Check sheet for the drawn part. Datum: minimum x, y, z corner. Units: mm. Give positions to 0.01 mm unless a question says otherwise; leave off trailing zeros. Write each loop counter-clockwise with the first axis right and the second up, starting at its lowest first coordinate (ties: lowest second). Pieces come first, ordered by that corner, then holes. Notation, with made-up numbers: (62.25, 8.25) -> (93.25, 8.25) arc R32 cw to (93.25, 44.25) -> close; hole circle Ø8 at (80.5, -3). An arc over 180 degrees is marked (long way). Answer as CSV lines item,"result". Start each with the question number.
1) Sectioned sample at D-D on x = 51.5. Record the cut outline in (y, z).
2) Sectioned sample at C-C on z = 41. Record the cut outline in (x, y), and give its area (3 significant figures).
3) Sectioned sample at A-A on y = 0.4. Give the number of separate pieces and of enclosed holes in the cut face, and give its area (3 significant figures).
4) Sectioned sample at B-B on z = 85.2. Record the cut outline in (x, y).
5) Material ranges on L1, parallel to Z at x = 85.2, y = 0.75; L2, parallel to X at y = 0.4, z = 85.2; L3, parallel to Z at x = 37, y = 1.1 (1 decimal), recorded low to high.
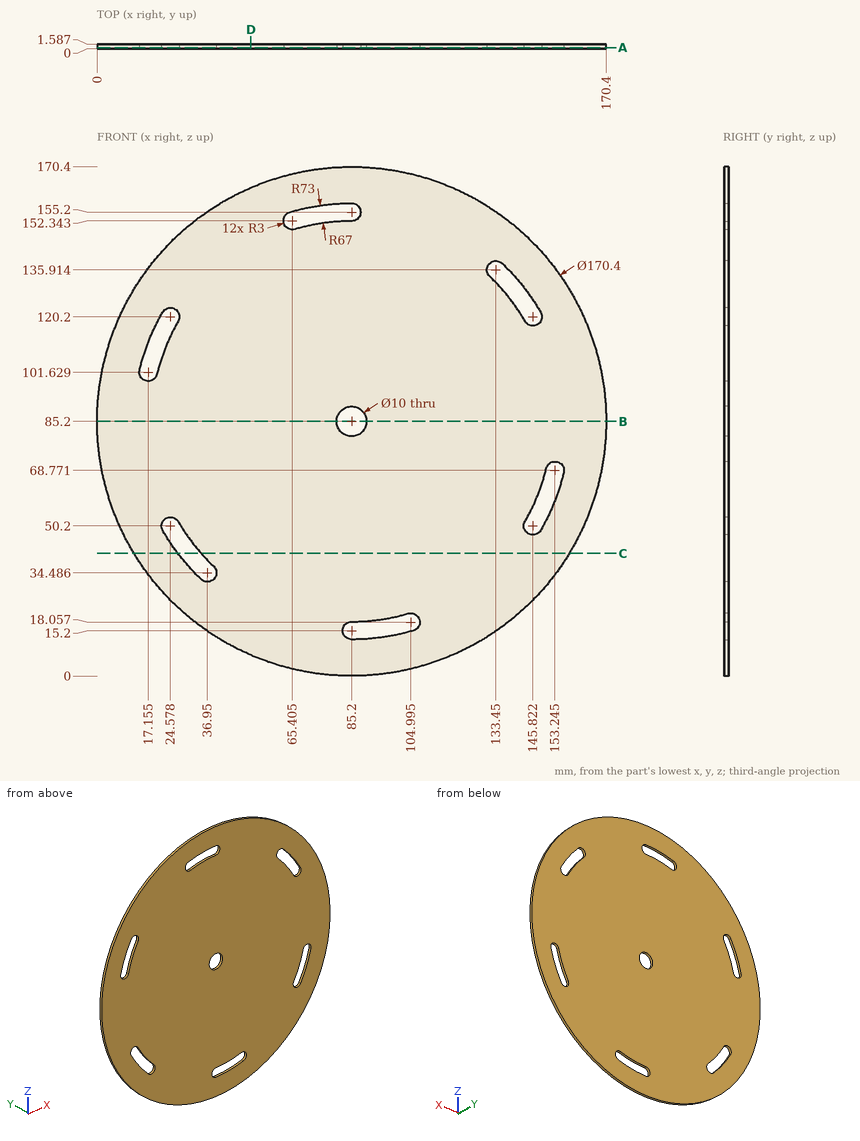
Ans:
1,outline,"(0, 6.95) -> (1.59, 6.95) -> (1.59, 163.45) -> (0, 163.45) -> close"
2,outline,"(12.36, 0) -> (27.1, 0) -> (27.1, 1.59) -> (12.36, 1.59) -> close; (34.85, 0) -> (158.04, 0) -> (158.04, 1.59) -> (34.85, 1.59) -> close"
2,area,"219 mm²"
3,separate pieces,"1"
3,enclosed holes,"7"
3,area,"21,800 mm²"
4,outline,"(0, 0) -> (80.2, 0) -> (80.2, 1.59) -> (0, 1.59) -> close; (90.2, 0) -> (170.4, 0) -> (170.4, 1.59) -> (90.2, 1.59) -> close"
5,L1,"z = 0 to 12.2, 18.2 to 80.2, 90.2 to 152.2, 158.2 to 170.4"
5,L2,"x = 0 to 80.2, 90.2 to 170.4"
5,L3,"z = 14.9 to 31.5, 38.7 to 155.5"
